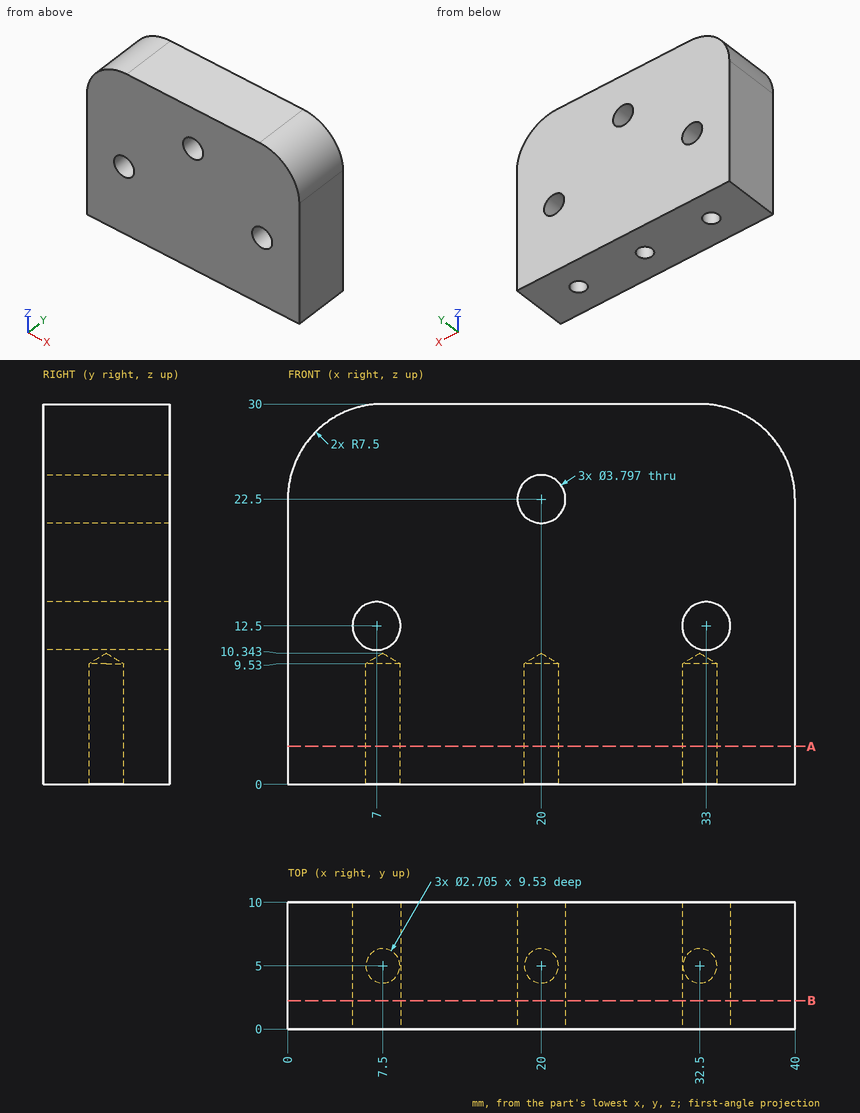
The figure shows three views and two pictorial views of one solid part (mm, origin at its lowest corner). Answer the questions. Round coordinates to 2 decimals unless told otherwise and drop trailing zeros. Order: outer loops, then holes, each group sorted by start corner. A loop starts at its lowest first (then second) coordinate and runs counter-clockwise, first axis right, second up. Notation, with made-up numbers: (66, -33) -> (115, -33) arc R30 cw to (115, 5) -> close; hole circle Ø5 at (64.5, 55). An arc over 180 degrees is marked (long way). Put each result on its own line as item: value.
Q1. Section B-B, the plane y = 2.25 is taken. Write down the section's boundary in (x, z).
Results list:
outline: (0, 0) -> (40, 0) -> (40, 22.5) arc R7.5 ccw to (32.5, 30) -> (7.5, 30) arc R7.5 ccw to (0, 22.5) -> close; hole circle Ø3.8 at (7, 12.5); hole circle Ø3.8 at (20, 22.5); hole circle Ø3.8 at (33, 12.5)
Q2. Section A-A, the plane z = 3 is taken. Write down the section's boundary in (x, y) (1 decimal).
Results list:
outline: (0, 0) -> (40, 0) -> (40, 10) -> (0, 10) -> close; hole circle Ø2.7 at (7.5, 5); hole circle Ø2.7 at (20, 5); hole circle Ø2.7 at (32.5, 5)
Q3. Consider line 1 along X through (y, z) = (5, 6.5); line 2 along Y through (x, z) = (32.5, 5.5); line 3 along X through (y, z) = (7, 12.5). Determine where each line is inside the solid, lowest interval first.
Results list:
line 1: 0 to 6.15, 8.85 to 18.65, 21.35 to 31.15, 33.85 to 40
line 2: 0 to 3.65, 6.35 to 10
line 3: 0 to 5.1, 8.9 to 31.1, 34.9 to 40
Q4. Each of these flat-tipped pins is pushed along its axis until it touches: P1, Ø5, axis at y = 4, z = 24.5, coming from the +X side; P2, Ø3, axis at x = 33, z = 12.5, coming from the -Y side; P3, Ø2, axis at x = 20, y = 5, coming from the -Z side. Where does it stop, or does it pass through?
Results list:
P1: x = 40
P2: through
P3: z = 9.74
